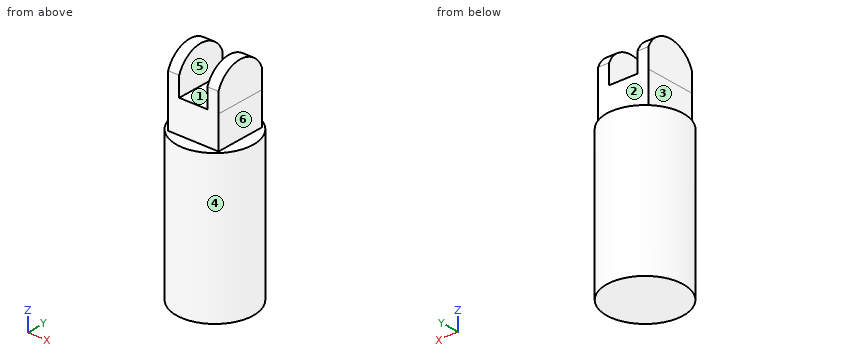
```python
from build123d import *

# Parameters (mm, degrees)
SKETCH1_R           = 6.475
BOSS_EXTRUDE1_DEPTH = 25
SKETCH5_W           = 8.55
SKETCH5_H           = 8.55
BOSS_EXTRUDE2_DEPTH = 5.5
SKETCH10_W          = 1.88
SKETCH10_H          = 8.55
BOSS_EXTRUDE3_DEPTH = 3.3
SKETCH8_W           = 1.88
SKETCH8_H           = 8.55
BOSS_EXTRUDE4_DEPTH = 3.3
BOSS_EXTRUDE5_DEPTH = 1.88
BOSS_EXTRUDE6_DEPTH = 1.88


with BuildPart() as part:
    # Sketch1 → Boss-Extrude1 (new body)
    with BuildSketch(Plane.XY):
        Circle(SKETCH1_R)
    extrude(amount=BOSS_EXTRUDE1_DEPTH)

    # Sketch5 → Boss-Extrude2 (add)
    with BuildSketch(Plane.XY.offset(25)):
        Rectangle(SKETCH5_W, SKETCH5_H)
    extrude(amount=BOSS_EXTRUDE2_DEPTH)

    # Sketch10 → Boss-Extrude3 (add)
    with BuildSketch(Plane.XY.offset(30.5)):
        with Locations((-3.322891498, 0)):
            Rectangle(SKETCH10_W, SKETCH10_H)
    extrude(amount=BOSS_EXTRUDE3_DEPTH)

    # Sketch8 → Boss-Extrude4 (add)
    with BuildSketch(Plane.XY.offset(30.5)):
        with Locations((3.335018839, 0)):
            Rectangle(SKETCH8_W, SKETCH8_H)
    extrude(amount=BOSS_EXTRUDE4_DEPTH)

    # Sketch11 → Boss-Extrude5 (add)
    with BuildSketch(Plane(origin=(4.275018839, 0, 0), x_dir=(0, 0, -1), z_dir=(1, 0, 0))):
        with BuildLine():
            Line((-33.8, 4.275), (-33.8, -4.275))
            ThreePointArc((-33.8, -4.275), (-36.736596519, 0), (-33.8, 4.275))
        make_face()
    extrude(amount=-BOSS_EXTRUDE5_DEPTH)

    # Sketch12 → Boss-Extrude6 (add)
    with BuildSketch(Plane.ZY.offset(4.262891498)):
        with BuildLine():
            Line((33.8, 4.275), (33.8, -4.275))
            ThreePointArc((33.8, -4.275), (36.736596519, 0), (33.8, 4.275))
        make_face()
    extrude(amount=-BOSS_EXTRUDE6_DEPTH)


solid = part.part
```
Design review of the part built by this model. Coordinates are the model's own, in mm. Face numbers are marked on the shaded views. A direction names the side the tool comes from. Give positions to 0.01 mm unless a question says otherwise; leave off trailing zeros. Order: outer loops, then holes, each group sorted by start corner. A loop starts at its lowest first (then second) coordinate and runs counter-clockwise, first axis right, second up. Notation, with made-up numbers: (74.5, 64) -> (95.5, 64) arc R17 ccw to (95.5, 78) -> close; hole circle Ø1 at (-39, 20.5). An arc over 180 degrees is marked (long way). Write item = value, one per line. Start each with the question number.
(1) We need section C-C on x = 0. Write out the cut boundary in (y, z) (3 decimals).
(2) For pin 1 (4 mm diameter, centred on y = -3.5, z = 16, fed in from +X); pin 2 (4.5 mm diameter, centred on x = -2, z = 31, fed in from +Y) (3 decimals); pin 3 (1.9 mm diameter, centred on y = -1.5, z = 32, fed in from +X) (3 decimals); pin 4 (1.5 mm diameter, centred on x = -1, z = 32, fed in from -Y), all flat-tipped, find the tip position at first contact; note any pin that passes through.
(3) We need section D-D on z = 21. Write out the cut boundary in (x, y) (3 decimals).
(4) To check wall thickness, follow line 1 along X through (y, z) = (-2.5, 25.5) (3 decimals); line 2 along Z through (x, y) = (-3, -4.75). State the ranges of each line that lie inside material, in increasing order.
(5) We need section A-A on z = 32.5. Write out the cut boundary in (x, y) (3 decimals), plus the area to 3 significant figures.
(6) Mouldability with a two-part tool opening along X and no side actions: class the marked faces 4, 5 and 6 as +X half, -X half, draft (parallel to the pull), parting line (faces both ways), or undercut.
(7) For the marked faces 1, 2 and 3, list the 3-axis set-ups (+Z, -Z, +X, -X, +Y, -Y) from which the entire face can be reached by the end or side of a thin tool; tool diameter is ignored.
Numbers:
q1.outline = (-6.475, 0) -> (6.475, 0) -> (6.475, 25) -> (4.275, 25) -> (4.275, 30.5) -> (-4.275, 30.5) -> (-4.275, 25) -> (-6.475, 25) -> close
q2.pin_1 = 6.3
q2.pin_2 = 4.275
q2.pin_3 = 4.275
q2.pin_4 = through
q3.outline = circle Ø12.95 at (0, 0)
q4.line_1 = -4.275 to 4.275
q4.line_2 = 0 to 25
q5.outline = (-4.263, -4.275) -> (-2.383, -4.275) -> (-2.383, 4.275) -> (-4.263, 4.275) -> close; (2.395, -4.275) -> (4.275, -4.275) -> (4.275, 4.275) -> (2.395, 4.275) -> close
q5.area = 32.1 mm^2
q6.face_4 = parting line
q6.face_5 = undercut
q6.face_6 = +X half
q7.face_1 = +Z, +Y, -Y
q7.face_2 = +Z, +X, -X, +Y
q7.face_3 = +Z, -X, +Y, -Y
